```python
from build123d import *

# Parameters (mm, degrees)
EXTRUDE_1_DEPTH      = 3
EXTRUDE_1_DEPTH_BACK = 3
SKETCH_1_R           = 64
EXTRUDE_2_DEPTH      = 4
EXTRUDE_2_DEPTH_BACK = 7
SKETCH_2_R           = 5
SKETCH_3_R           = 2.5
CUT_EXTRUDE_1_DEPTH  = 92.175654645


with BuildPart() as part:
    # Sketch 1 → Extrude 1 (new, two sides: drawn at the far end of the back side and taken through both)
    with BuildSketch(Plane(origin=(0, 0, 0), x_dir=(1, 0, 0), z_dir=(0, 1, 0)).offset(-EXTRUDE_1_DEPTH_BACK)):
        with Locations(Location((0, 0, 0), (0, 0, 270))):
            Circle(SKETCH_1_R)
    extrude(amount=EXTRUDE_1_DEPTH + EXTRUDE_1_DEPTH_BACK)

    # Sketch 2 → Extrude 2 (add, two sides: drawn at the far end of the back side and taken through both)
    with BuildSketch(Plane(origin=(0, 0, 0), x_dir=(1, 0, 0), z_dir=(0, 1, 0)).offset(-EXTRUDE_2_DEPTH_BACK)):
        with Locations(Location((0, 0, 0), (0, 0, 270))):
            Circle(SKETCH_2_R)
    extrude(amount=EXTRUDE_2_DEPTH + EXTRUDE_2_DEPTH_BACK)

    # Sketch 3 → Cut-Extrude 1 (cut, through all)
    with BuildSketch(Plane(origin=(0, 4, 0), x_dir=(1, 0, 0), z_dir=(0, 1, 0))):
        with Locations(Location((0, 0, 0), (0, 0, 270))):
            Circle(SKETCH_3_R)
    extrude(amount=-CUT_EXTRUDE_1_DEPTH, mode=Mode.SUBTRACT)


solid = part.part
```
The listing builds one solid part. Answer for the finished solid, in the listing's coordinates (mm). A direction names the side the tool comes from. Coordinates: 2 decimals unless noted, no trailing zeros. Write each loop counter-clockwise with the first axis right and the second up, starting at its lowest first coordinate (ties: lowest second). Pieces come first, ordered by that corner, then holes. Notation, with made-up numbers: (54, 66) - (81, 66) arc R32 cw to (81, 93) - close; hole circle Ø6 at (57.5, 18). An arc over 180 degrees is marked (long way). Return JSON: item names as keys, results as strings. Group by question number.
1. Determine the mould class of faces 1 (the cylindrical face through (-2.44, -1.42, -0.54)), 2 (the flat face through (-2, -7, 2)), 3 (the cylindrical face through (-4.88, 3.49, -1.08)) for opening direction Z: released by +Z, released by -Z, zero draft, split by the parting line, or undercut.
2. A cutting plane is placed at D-D, the plane z = -56. Determine the outline of the cut face in (x, y).
3. A cutting plane is placed at C-C, the plane y = -5.25. Determine the outline of the cut face in (x, z), plus the area to 3 significant figures.
4. Which of the six approach directions +Z, -Z, +X, -X, +Y, -Y give full straight-line access (tool end or side, diameter ignored) to faces 4 (the cylindrical face through (-62.48, -0.04, -13.87)), 5 (the cylindrical face through (-4.88, -5.03, -1.08))?
5. Given pin 1 (1.5 mm diameter, centred on x = 38, z = -44.5, fed in from -Y); pin 2 (6 mm diameter, centred on x = 0, z = 0, fed in from -Y); pin 3 (1.5 mm diameter, centred on y = 2, z = -17.5, fed in from +X); pin 4 (3 mm diameter, centred on x = 26.5, y = 0.5, fed in from -Z), each flat-ended and moving along its own axis, determine where each tip first touches the part or whether it passes through.
6. A cutting plane is placed at A-A, the plane z = 0. Determine the outline of the cut face in (x, y), plus the area to 3 significant figures.
7. A cutting plane is placed at B-B, the plane x = 0. Determine the outline of the cut face in (y, z), plus the area to 3 significant figures.
8. Straight lines are drawn through the part: L1, parallel to Y at x = 32.5, z = -26; L2, parallel to X at y = 1, z = 0; L3, parallel to Z at x = 26.5, y = 1.5. For each, find the intervals that lie inside material, in ascending order.
Ans:
{
 "1": {"face 1": "undercut", "face 2": "zero draft", "face 3": "split by the parting line"},
 "2": {"outline": "(-30.98, -3) - (30.98, -3) - (30.98, 3) - (-30.98, 3) - close"},
 "3": {"outline": "circle Ø10 at (0, 0); hole circle Ø5 at (0, 0)", "area": "58.9 mm²"},
 "4": {"face 4": "+Y, -Y", "face 5": "-Y"},
 "5": {"pin 1": "y = -3", "pin 2": "y = -7", "pin 3": "x = 61.77", "pin 4": "z = -58.92"},
 "6": {"outline": "(-64, -3) - (-5, -3) - (-5, -7) - (-2.5, -7) - (-2.5, 4) - (-5, 4) - (-5, 3) - (-64, 3) - close; (2.5, -7) - (5, -7) - (5, -3) - (64, -3) - (64, 3) - (5, 3) - (5, 4) - (2.5, 4) - close", "area": "763 mm²"},
 "7": {"outline": "(-7, -5) - (-3, -5) - (-3, -64) - (3, -64) - (3, -5) - (4, -5) - (4, -2.5) - (-7, -2.5) - close; (-7, 2.5) - (4, 2.5) - (4, 5) - (3, 5) - (3, 64) - (-3, 64) - (-3, 5) - (-7, 5) - close", "area": "763 mm²"},
 "8": {"L1": "-3 to 3", "L2": "-64 to -2.5, 2.5 to 64", "L3": "-58.26 to 58.26"}
}
